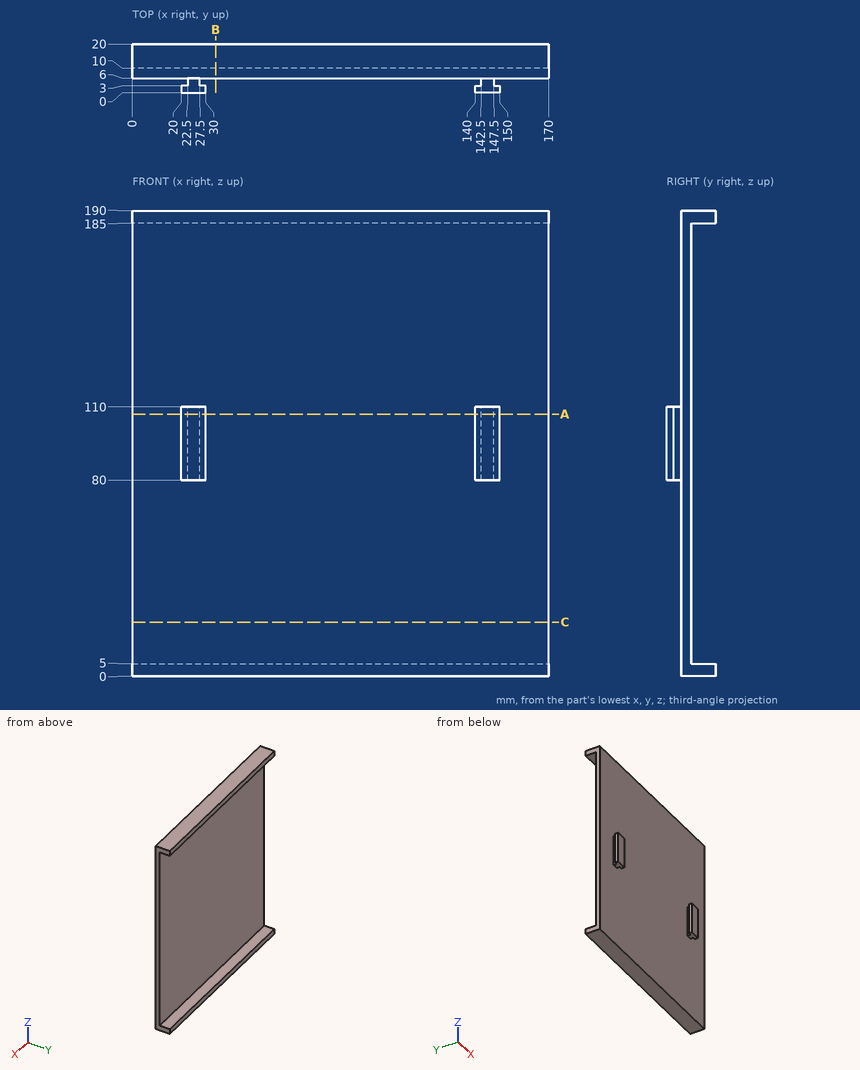
Geometry: see drawing. Coordinates: mm, zero at the bounding-box minimum. Round coordinates to 2 decimals unless told otherwise and drop trailing zeros. Write each loop counter-clockwise with the first axis right and the second up, starting at its lowest first coordinate (ties: lowest second). Pieces come first, ordered by that corner, then holes. Notation, with made-up numbers: (89, 4.5) - (135, 4.5) arc R26 ccw to (135, 31.5) - close; hole circle Ø7 at (15, 89.5). An arc over 180 degrees is marked (long way). Use CSV: the item, a comma, the result in double quotes. Start each with the question number.
(1) Cut plane A-A, the plane z = 107. Return loops of the section in (x, y).
(2) Cut plane C-C, the plane z = 22. Return loops of the section in (x, y).
(3) First-contact query: pin 1 Ø3.5 at (y, z) = (1.5, 98.5) entering from +X; pin 2 Ø1.2 at (x, z) = (141.5, 100.5) entering from +Y; pin 3 Ø8 at (x, z) = (135, 164.5) entering from -Y. Flat tips, straight axial feed; report the tip coordinate or a pass-through.
(4) Cut plane B-B, the plane x = 34. Return loops of the section in (y, z), and give its area (3 significant figures).
(5) Material intervals for probe 1 along Z at (x, y) = (122, 19); probe 2 along X at (y, z) = (1.75, 95.5); probe 3 along Y at (x, z) = (65.5, 85), sorted ascending. Write a range as [from, to].
Geometry says:
1,outline,"(0, 6) - (22.5, 6) - (22.5, 3) - (20, 3) - (20, 0) - (30, 0) - (30, 3) - (27.5, 3) - (27.5, 6) - (142.5, 6) - (142.5, 3) - (140, 3) - (140, 0) - (150, 0) - (150, 3) - (147.5, 3) - (147.5, 6) - (170, 6) - (170, 10) - (0, 10) - close"
2,outline,"(0, 6) - (170, 6) - (170, 10) - (0, 10) - close"
3,pin 1,"x = 150"
3,pin 2,"y = 10"
3,pin 3,"y = 6"
4,outline,"(6, 0) - (20, 0) - (20, 5) - (10, 5) - (10, 185) - (20, 185) - (20, 190) - (6, 190) - close"
4,area,"860 mm²"
5,probe 1,"[0, 5], [185, 190]"
5,probe 2,"[20, 30], [140, 150]"
5,probe 3,"[6, 10]"
